Study the drawing (mm; zero at the part's minimum x, y, z) and answer. A direction names the side the tool comes from. Give positions to 0.01 mm unless a question says otherwise; leave off trailing zeros. Write each loop counter-clockwise with the first axis right and the second up, starting at its lowest first coordinate (ties: lowest second). Pieces come first, ordered by that corner, then holes. Notation, with made-up numbers: (20.5, 58.25) - (29.5, 58.25) arc R31 cw to (29.5, 94.25) - close; hole circle Ø6 at (-35.5, 35). An arc over 180 degrees is marked (long way). Return JSON: item names as keys, results as strings.
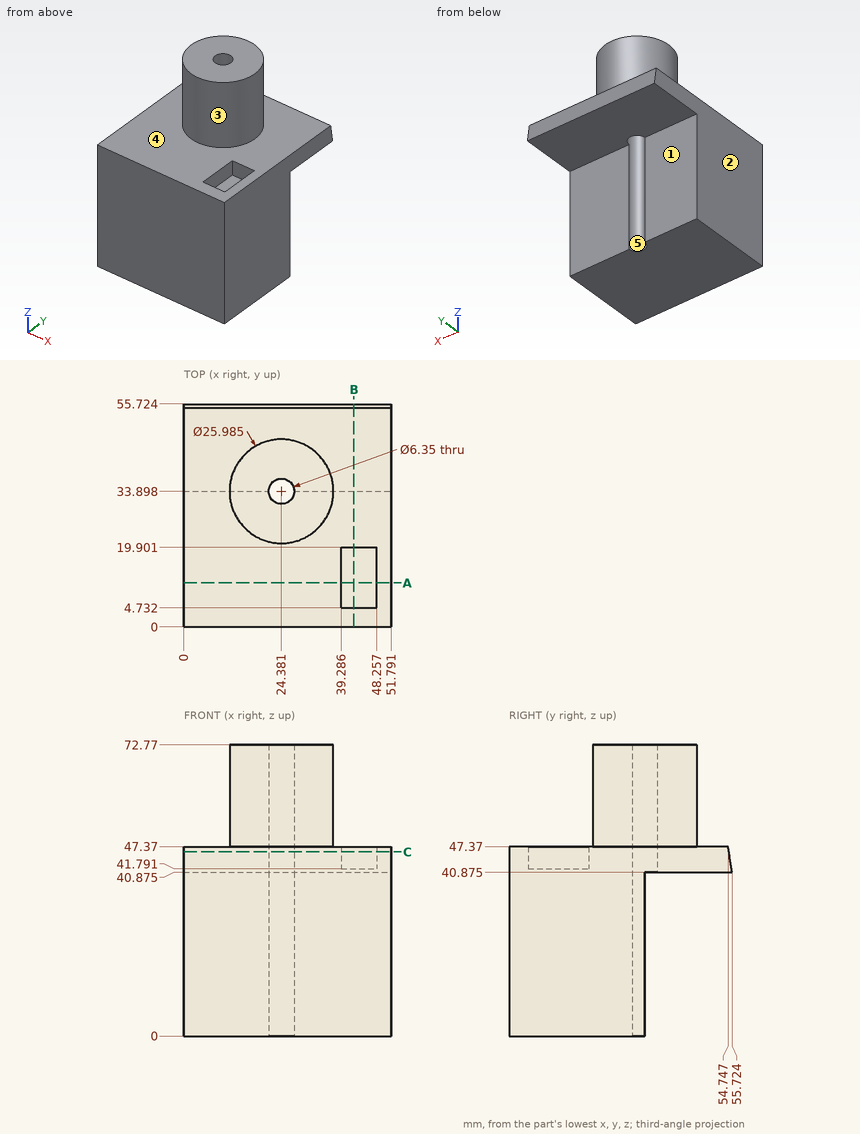
Item 1: The mould has two halves that part along Y. Classify the marked faces 3, 4 and 5: +Y half, -Y half, draft (parallel to the pull), parting line (faces both ways), or undercut.
Answer below:
{"face 3": "parting line", "face 4": "draft", "face 5": "undercut"}
Item 2: Consider L1, parallel to Z at x = 23.5, y = 19; L2, parallel to Y at x = 14, z = 15; L3, parallel to Z at x = 23, y = 47 (1 decimal). Determine where each line is inside the solid, lowest interval first.
Answer below:
{"L1": "z = 0 to 47.37", "L2": "y = 0 to 33.9", "L3": "z = 40.9 to 47.4"}
Item 3: A cutting plane is placed at C-C on z = 46. Give the number of separate pieces and of enclosed holes in the cut face, then the cut area to 3 significant figures.
Answer below:
{"separate pieces": "1", "enclosed holes": "2", "area": "2,680 mm²"}
Item 4: Flat-ended cylindrical pins translate along their axes: P1, Ø1.7, axis at x = 42.5, z = 43.5, coming from the +Y side; P2, Ø10.5, axis at x = 11, z = 21.5, coming from the +Y side; P3, Ø6, axis at x = 17.5, y = 45.5, coming from the -Z side (1 decimal); P4, Ø4, axis at x = 24.38, y = 33.9, coming from the +Z side. Find the tip coordinate at first contact, or state that the pin passes through.
Answer below:
{"P1": "stops at y = 55.46", "P2": "stops at y = 33.9", "P3": "stops at z = 40.9", "P4": "passes through"}
Item 5: A cutting plane is placed at B-B on x = 42.5. Determine the outline of the cut face in (y, z) (1 decimal).
Answer below:
{"outline": "(0, 0) - (33.9, 0) - (33.9, 40.9) - (55.7, 40.9) - (54.7, 47.4) - (19.9, 47.4) - (19.9, 41.8) - (4.7, 41.8) - (4.7, 47.4) - (0, 47.4) - close"}
Item 6: A cutting plane is placed at A-A on y = 11. Determine the outline of the cut face in (x, z) (1 decimal), then the cut area to 3 significant figures.
Answer below:
{"outline": "(0, 0) - (51.8, 0) - (51.8, 47.4) - (48.3, 47.4) - (48.3, 41.8) - (39.3, 41.8) - (39.3, 47.4) - (0, 47.4) - close", "area": "2,400 mm²"}
Item 7: For the marked faces 1 and 2, determine the directions among +Z, -Z, +X, -X, +Y, -Y from which every point of the face is accessible in a straight line to the end or side of a thin tool.
Answer below:
{"face 1": "-Z, +X, -X, +Y", "face 2": "+Z, -Z, -X, +Y, -Y"}
